Geometry check sheet. Reference: drawing and pictorial views, mm from the part's lowest x, y, z. Coordinates: 2 decimals unless noted, no trailing zeros. Write each loop counter-clockwise with the first axis right and the second up, starting at its lowest first coordinate (ties: lowest second). Pieces come first, ordered by that corner, then holes. Notation, with made-up numbers: M 33,8.25 L 41,8.25 A19 cw 41,24.25 Z; hole C -19.75,-31 d10. An arc over 180 degrees is marked long. One line per item, written item: value.
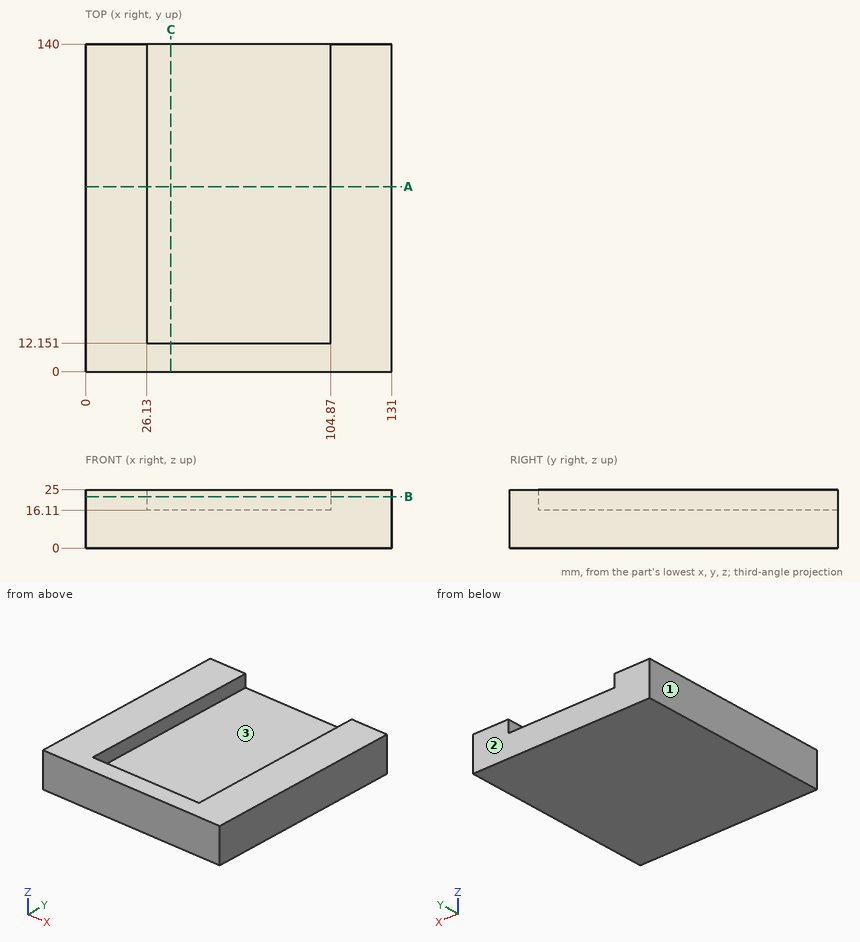
Item 1: Cross-section at C-C, the plane x = 36.5. Enter the section's corners in (y, z).
The answers:
outline: M 0,0 L 140,0 L 140,16.11 L 12.15,16.11 L 12.15,25 L 0,25 Z
Item 2: Cross-section at B-B, the plane z = 22. Enter the section's corners in (x, y).
The answers:
outline: M 0,0 L 131,0 L 131,140 L 104.87,140 L 104.87,12.15 L 26.13,12.15 L 26.13,140 L 0,140 Z
Item 3: Draft check along X on the marked faces 1, 2 and 3. Enter one of: released by +X, released by -X, zero draft, split by the parting line, or undercut.
The answers:
face 1: released by -X
face 2: zero draft
face 3: undercut
Item 4: Scan lines: line 1 (X direction, y = 69.5, z = 18); line 2 (Y direction, x = 68.5, z = 19.75); line 3 (Z direction, x = 97.5, y = 31). Record each from-to range of solid material in increasing order.
The answers:
line 1: x = 0 to 26.13, 104.87 to 131
line 2: y = 0 to 12.15
line 3: z = 0 to 16.11
Item 5: Go/stop test with flat-tipped pins: P1, Ø10, axis at y = 86, z = 20, coming from the -X side; P2, Ø7, axis at x = 61.5, z = 20.5, coming from the +Y side. Record where each tip stops, or that it passes through.
The answers:
P1: stops at x = 0
P2: stops at y = 12.15
Item 6: Cross-section at A-A, the plane y = 79. Enter the section's corners in (x, z), and give its area (4 significant figures).
The answers:
outline: M 0,0 L 131,0 L 131,25 L 104.87,25 L 104.87,16.11 L 26.13,16.11 L 26.13,25 L 0,25 Z
area: 2,575 mm²
